Verification items for the finished model (mm, model axes). Face numbers are marked on the shaded views. A direction names the side the tool comes from. Coordinates: 2 decimals unless noted, no trailing zeros. Loops run counter-clockwise (first coordinate to the right, second up) from the corner with the lowest first, then second, coordinate; pieces in that order, holes last. Notation, with made-up numbers: (-31.75, 57) -> (-4.75, 57) arc R23 cw to (-4.75, 91) -> close; hole circle Ø4 at (-11.5, 56.25). An arc over 180 degrees is marked (long way). Answer as a JSON object with one key per item and string values. Group by question number.
Q1. Release check for a two-part mould opening along X. For the marked faces 5, 6 and 7 record: released by +X, released by -X, zero draft, split by the parting line, or undercut.
Q2. Cross-section at A-A on z = -8.25. Record the boundary of the cut face in (x, y), and give its area (3 significant figures).
Q3. Scan lines: L1, parallel to X at y = -1.25, z = -9.5; L2, parallel to X at y = 10, z = 2.5; L3, parallel to Z at x = 11.25, y = 7.5. Record each from-to range of solid material in increasing order.
Q4. Set-up check for the marked faces 1, 2, 3 and 4: record each of +Z, -Z, +X, -X, +Y, -Y from which the full face is reachable in a straight line by a thin tool's end or side.
Q5. Gauge pin test, flat ends, axial feed: pin 1 Ø4.5 at (x, y) = (0, 0) entering from -Z; pin 2 Ø5 at (x, z) = (0.5, -9) entering from +Y; pin 3 Ø1.8 at (x, z) = (0.5, -8.5) entering from -Y. Record the tip position at first contact, or that the pin passes through.
Q6. Cross-section at B-B on y = -11. Give the number of separate pieces and of enclosed holes in the cut face, and give its area (3 significant figures).
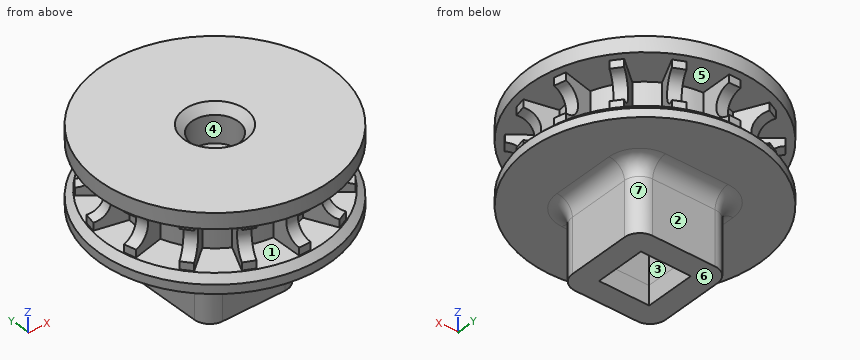
```python
from build123d import *

# Parameters (mm, degrees)
EXTRUDE_1_DEPTH          = 0.75
PATTERN_CIRCULAR_1_COUNT = 14
SKETCH_3_W               = 6.1
SKETCH_3_H               = 6.1
EXTRUDE_2_DEPTH          = 9
FILLET_1_R               = 2
CHAMFER_1_SIZE           = 0.2
CHAMFER_1_SIZE2          = 2.286010461
SKETCH_4_R               = 1.75
CUT_EXTRUDE_1_DEPTH      = 29.478061732
SKETCH_6_R               = 3
CUT_EXTRUDE_2_DEPTH      = 6
CHAMFER_2_SIZE           = 1
CHAMFER_3_SIZE           = 1.5
CHAMFER_4_SIZE           = 0.85


with BuildPart() as part:
    # 草圖1 → 旋轉1 (revolve)
    with BuildSketch(Plane(origin=(0, 0, 0), x_dir=(0, 0, -1), z_dir=(1, 0, 0)), mode=Mode.PRIVATE) as revolve_1_sk:
        Polygon((-5, 0), (5, 0), (5, 15), (3, 15), (3, 10), (-3, 10), (-3, 15), (-5, 15), align=None)
    revolve(revolve_1_sk.sketch.rotate(Axis((0, 0, 5), (0, 0, -1)), 90), axis=Axis((0, 0, 5), (0, 0, -1)))

    # 草圖2 → 填料-伸長1 (add, symmetric)
    with BuildSketch(Plane(origin=(0, 0, 0), x_dir=(0, 0, -1), z_dir=(1, 0, 0))):
        with BuildLine():
            Line((3, 10), (3, 14))
            Line((3, 14), (2, 14))
            ThreePointArc((2, 14), (0, 12), (-2, 14))
            Line((-2, 14), (-3, 14))
            Line((-3, 14), (-3, 10))
            Line((-3, 10), (-3, 8.5))
            Line((-3, 8.5), (3, 8.5))
            Line((3, 8.5), (3, 10))
        make_face()
    extrude_1 = extrude(amount=EXTRUDE_1_DEPTH, both=True)

    # 環狀複製排列1: 填料-伸長1 ×14 about axis
    pattern_circular_1_axis = Axis((0, 0, 0), (0, 0, 1))
    for i in range(1, PATTERN_CIRCULAR_1_COUNT):
        add(extrude_1.rotate(pattern_circular_1_axis, i * 360 / PATTERN_CIRCULAR_1_COUNT))

    # 草圖3 → 填料-伸長2 (add)
    with BuildSketch(Plane(origin=(0, 0, -5), x_dir=(-1, 0, 0), z_dir=(0, 0, -1))):
        with BuildLine():
            Line((-4.05, -6.05), (4.05, -6.05))
            ThreePointArc((4.05, -6.05), (5.464213562, -5.464213562), (6.05, -4.05))
            Line((6.05, -4.05), (6.05, 4.05))
            ThreePointArc((6.05, 4.05), (5.464213562, 5.464213562), (4.05, 6.05))
            Line((4.05, 6.05), (-4.05, 6.05))
            ThreePointArc((-4.05, 6.05), (-5.464213562, 5.464213562), (-6.05, 4.05))
            Line((-6.05, 4.05), (-6.05, -4.05))
            ThreePointArc((-6.05, -4.05), (-5.464213562, -5.464213562), (-4.05, -6.05))
        make_face()
        Rectangle(SKETCH_3_W, SKETCH_3_H, mode=Mode.SUBTRACT)
    extrude(amount=EXTRUDE_2_DEPTH)

    # 圓角1
    fillet_1_edges = [part.edges().sort_by_distance(p)[0] for p in [
        (5.464213562, -5.464213562, -5),
        (0, -6.05, -5),
        (-5.464213562, -5.464213562, -5),
        (-6.05, 0, -5),
        (-5.464213562, 5.464213562, -5),
        (0, 6.05, -5),
        (5.464213562, 5.464213562, -5),
        (6.05, 0, -5),
    ]]
    fillet(fillet_1_edges, radius=FILLET_1_R)

    # 導角1
    chamfer_1_edges = [part.edges().sort_by_distance(p)[0] for p in [
        (-3.05, 0, -14),
        (0, 3.05, -14),
        (3.05, 0, -14),
        (0, -3.05, -14),
    ]]
    chamfer_1_side = [part.faces().sort_by_distance(p)[0] for p in [
        (5.343213562, -5.343213562, -14),
    ]]
    chamfer(chamfer_1_edges, length=CHAMFER_1_SIZE, length2=CHAMFER_1_SIZE2, reference=chamfer_1_side[0])

    # 草圖4 → 除料-伸長1 (cut, through all)
    with BuildSketch(Plane.XY.offset(5)):
        Circle(SKETCH_4_R)
    extrude(amount=-CUT_EXTRUDE_1_DEPTH, mode=Mode.SUBTRACT)

    # 草圖6 → 除料-伸長2 (cut)
    with BuildSketch(Plane.XY.offset(5)):
        Circle(SKETCH_6_R)
    extrude(amount=-CUT_EXTRUDE_2_DEPTH, mode=Mode.SUBTRACT)

    # 導角2
    chamfer_2_edges = [part.edges().sort_by_distance(p)[0] for p in [
        (-3, 0, 5),
    ]]
    chamfer(chamfer_2_edges, length=CHAMFER_2_SIZE)

    # 導角3
    # the kernel refuses this chamfer: 1.5 mm, written as the material it adds along each edge
    with BuildSketch(Plane(origin=(0, 0, -1), x_dir=(1, 0, 0), z_dir=(0, -1, 0))) as chamfer_3_piece_1_section:
        Polygon((3, CHAMFER_3_SIZE), (3 - CHAMFER_3_SIZE, 0), (3, 0), align=None)
    chamfer_3_piece_1 = revolve(axis=Axis((0, 0, -1), (0, 0, 1)), mode=Mode.PRIVATE)
    chamfer_3_piece_1 = chamfer_3_piece_1 - Plane(origin=(0, 0, -0.122651597), x_dir=(1, 0, 0), z_dir=(0, 0, 1)) * Cylinder(1.75, 12, mode=Mode.PRIVATE)
    add(chamfer_3_piece_1)

    # 導角4
    chamfer_4_edges = [part.edges().sort_by_distance(p)[0] for p in [
        (-15, 0, -3),
    ]]
    chamfer(chamfer_4_edges, length=CHAMFER_4_SIZE)


solid = part.part
```
Computed values:
{
 "1": {"face 5": "undercut", "face 6": "zero draft", "face 7": "released by +X"},
 "2": {"outline": "(-6.05, -4.05) arc R2 ccw to (-4.05, -6.05) -> (4.05, -6.05) arc R2 ccw to (6.05, -4.05) -> (6.05, 4.05) arc R2 ccw to (4.05, 6.05) -> (-4.05, 6.05) arc R2 ccw to (-6.05, 4.05) -> close; hole (-3.05, -3.05) -> (3.05, -3.05) -> (3.05, 3.05) -> (-3.05, 3.05) -> close", "area": "106 mm²"},
 "3": {"L1": "x = -6.05 to -3.05, 3.05 to 6.05", "L2": "x = -5.65 to -3.98, -0.75 to 0.75, 3.98 to 5.65", "L3": "z = -5 to -3, 3 to 5"},
 "4": {"face 1": "none", "face 2": "-Z, +X, -X, +Y", "face 3": "-Z", "face 4": "+Z"},
 "5": {"pin 1": "stops at z = -5", "pin 2": "stops at y = 6.11", "pin 3": "stops at y = -6.05"},
 "6": {"separate pieces": "1", "enclosed holes": "2", "area": "104 mm²"}
}
